Study the drawing (mm; zero at the part's minimum x, y, z) and answer. A direction names the side the tool comes from. Give positions to 0.01 mm unless a question says otherwise; leave off trailing zeros. Order: outer loops, then holes, each group sorted by start corner. A loop starts at its lowest first (then second) coordinate and runs counter-clockwise, first axis right, second up. Notation, with made-up numbers: (-12.75, -22) - (-0.75, -22) arc R3 cw to (-0.75, -18) - close; hole circle Ø6 at (-22, 42.25). An arc over 180 degrees is marked (long way). Put each result on its own line as item: value.
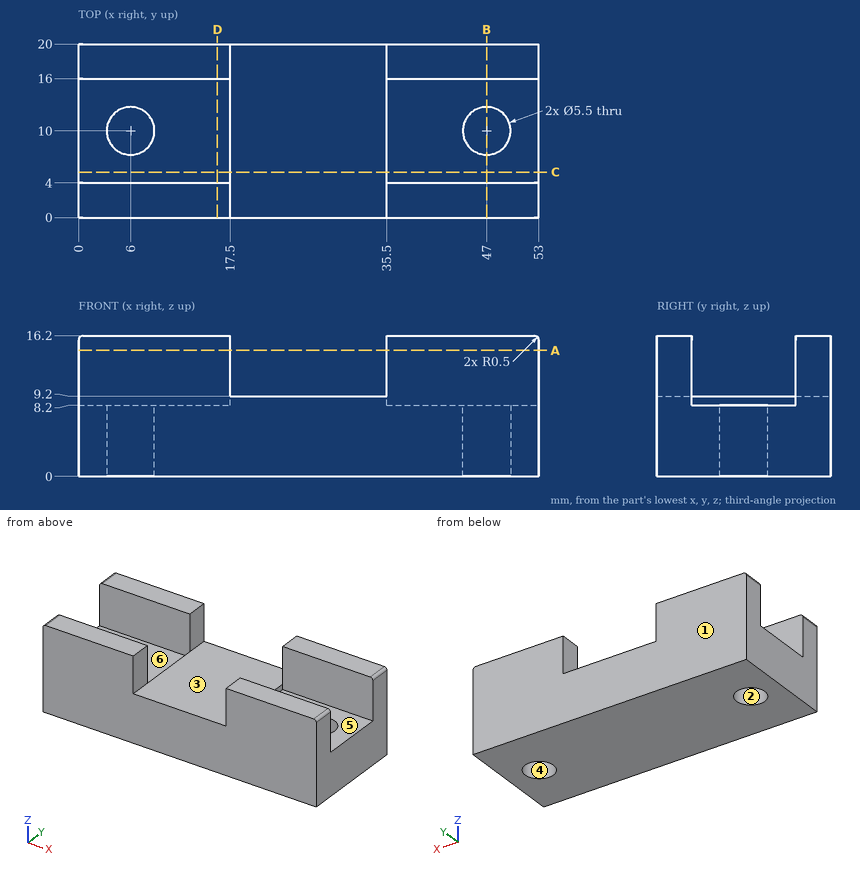
(1) Section B-B, the plane x = 47 is taken. Write down the section's boundary in (y, z).
Geometry check:
outline: (0, 0) - (7.25, 0) - (7.25, 8.2) - (4, 8.2) - (4, 16.2) - (0, 16.2) - close; (12.75, 0) - (20, 0) - (20, 16.2) - (16, 16.2) - (16, 8.2) - (12.75, 8.2) - close
(2) Straight lines are drawn through the part: line 1 (Y direction, x = 6, z = 2); line 2 (X direction, y = 2.75, z = 13.25); line 3 (Z direction, x = 4, y = 7.5). For each, find the intervals that lie inside material, in ascending order.
Geometry check:
line 1: y = 0 to 7.25, 12.75 to 20
line 2: x = 0 to 17.5, 35.5 to 53
line 3: z = 0 to 8.2
(3) Determine the mould class of the marked faces 1, 2 and 3 for opening direction Y: pulls with the +Y half, pulls with the -Y half, needs draft (parallel to the pull), parting line crosses it, or undercut.
Geometry check:
face 1: pulls with the +Y half
face 2: undercut
face 3: needs draft
(4) Given pin 1 (9.5 mm diameter, centred on x = 47, y = 9, fed in from +Z); pin 2 (0.5 mm diameter, centred on y = 9.5, z = 9, fed in from -X); pin 3 (3.5 mm diameter, centred on x = 6, y = 10, fed in from +Z), each flat-ended and moving along its own axis, determine where each tip first touches the part or whether it passes through.
Geometry check:
pin 1: stops at z = 8.2
pin 2: stops at x = 17.5
pin 3: passes through
(5) Section A-A, the plane z = 14.5 is taken. Write down the section's boundary in (x, y).
Geometry check:
outline: (0, 0) - (17.5, 0) - (17.5, 4) - (0, 4) - close; (0, 16) - (17.5, 16) - (17.5, 20) - (0, 20) - close; (35.5, 0) - (53, 0) - (53, 4) - (35.5, 4) - close; (35.5, 16) - (53, 16) - (53, 20) - (35.5, 20) - close
(6) A tool of negligible diameter and unlimited length cuts with its end or side. For the marked faces 4, 5 and 6, from which of +Z, -Z, +X, -X, +Y, -Y can it reach the whole face along a straight path? Write none if from no direction.
Geometry check:
face 4: +Z, -Z
face 5: +Z, +X
face 6: +Z, -X
(7) Section C-C, the plane y = 5.25 is taken. Write down the section's boundary in (x, z).
Geometry check:
outline: (0, 0) - (53, 0) - (53, 8.2) - (35.5, 8.2) - (35.5, 9.2) - (17.5, 9.2) - (17.5, 8.2) - (0, 8.2) - close
(8) Section D-D, the plane x = 16 is taken. Write down the section's boundary in (y, z), then the cut area to 3 significant figures.
Geometry check:
outline: (0, 0) - (20, 0) - (20, 16.2) - (16, 16.2) - (16, 8.2) - (4, 8.2) - (4, 16.2) - (0, 16.2) - close
area: 228 mm²
